CAD build for the part. Positions are in the model's coordinates, mm. A direction names the side the tool comes from. Round coordinates to 2 decimals unless told otherwise and drop trailing zeros. Loops run counter-clockwise (first coordinate to the right, second up) from the corner with the lowest first, then second, coordinate; pieces in that order, holes last.
from build123d import *

# Parameters (mm, degrees)
BASEHEAD_DEPTH  = 7.68
SKETCH3_R       = 6
BASEBODY_DEPTH  = 50
CHAMFER1_SIZE   = 0.947
SLOT_DEPTH      = 60.735123043
SLOT_DEPTH_BACK = 60.735123043
SKETCH5_W       = 3
SKETCH5_H       = 3


with BuildPart() as part:
    # Sketch-BaseHead → BaseHead (new body)
    with BuildSketch(Plane(origin=(0, 0, 0), x_dir=(0, 0, -1), z_dir=(1, 0, 0))):
        Polygon((5.118210136, -8.865), (10.236420273, 0), (5.118210136, 8.865), (-5.118210136, 8.865), (-10.236420273, 0), (-5.118210136, -8.865), align=None)
    extrude(amount=BASEHEAD_DEPTH)

    # Sketch1 → Revolve1 (revolve)
    with BuildSketch(Plane.XY, mode=Mode.PRIVATE) as revolve1_sk:
        Polygon((7.68, 0), (8.18, 0), (8.18, -8.315), (7.68, -8.865), align=None)
    revolve(revolve1_sk.sketch.rotate(Axis((-4.001564945, 0, 0), (1, 0, 0)), 270), axis=Axis((-4.001564945, 0, 0), (1, 0, 0)))

    # Sketch3 → BaseBody (add)
    with BuildSketch(Plane(origin=(8.18, 0, 0), x_dir=(0, 0, -1), z_dir=(1, 0, 0))):
        Circle(SKETCH3_R)
    extrude(amount=BASEBODY_DEPTH)

    # Chamfer1
    chamfer1_edges = [part.edges().sort_by_distance(p)[0] for p in [
        (58.18, 0, 6),
    ]]
    chamfer(chamfer1_edges, length=CHAMFER1_SIZE)

    # Sketch4 → HeadChamfer (revolve, cut)
    with BuildSketch(Plane(origin=(-0.264637255, 0, 5.916896391), x_dir=(0, 0, -1), z_dir=(0, 1, 0))):
        Polygon((16.153316664, -0.264637255), (14.781896391, -0.264637255), (16.153316664, -0.763793413), align=None)
    revolve(axis=Axis((-4.001564945, 0, 0), (1, 0, 0)), mode=Mode.SUBTRACT)

    # Sketch5 → Slot (cut, two sides: drawn at the far end of the back side and taken through both)
    with BuildSketch(Plane(origin=(0, 0, 0), x_dir=(1, 0, 0), z_dir=(0, 1, 0)).offset(-SLOT_DEPTH_BACK)):
        with Locations((1.5, 0)):
            Rectangle(SKETCH5_W, SKETCH5_H)
    extrude(amount=SLOT_DEPTH + SLOT_DEPTH_BACK, mode=Mode.SUBTRACT)


solid = part.part
Item 1: Wall check: L1, parallel to X at y = 3.5, z = -7.25; L2, parallel to X at y = -8, z = 0.25; L3, parallel to Y at x = 26.5, z = 0. Give the ranges that are in metal, low to high.
Verdict:
L1: x = 0 to 8.18
L2: x = 3 to 8.18
L3: y = -6 to 6
Item 2: Mould opens along Z. For faces 1 (the conical face through (0.087, -7.973, -4.392)), 2 (the flat face through (3, 0, 0)), 3 (the flat face through (7.68, 0, 9.2)) say: released by +Z, released by -Z, zero draft, split by the parting line, or undercut.
Verdict:
face 1: released by -Z
face 2: undercut
face 3: zero draft
Item 3: Flat gauge pins, fed straight in: P1, Ø3, axis at x = 6.5, z = 8, coming from the +Y side; P2, Ø0.8, axis at y = 1, z = 9, coming from the +X side; P3, Ø2, axis at y = 6.5, z = 4.5, coming from the +X side; P4, Ø3.5, axis at y = 2.5, z = 0, coming from the -X side. Where does each tip first touch, or does it go through?
Verdict:
P1: stops at y = 6.47
P2: stops at x = 7.87
P3: stops at x = 8.18
P4: stops at x = 0
Item 4: Cut at A-A (x = 10.5). List the corners of the cut face in (y, z).
Verdict:
outline: circle Ø12 at (0, 0)
Item 5: 3-axis set-ups, long thin cutter, end or side, ignore diameter. For faces 4 (the flat face through (1, 0, 1.5)), 5 (the flat face through (7.68, -8, -5)), 6 (the flat face through (7.68, -8, 4.4)): which of +Z, -Z, +X, -X, +Y, -Y reach the whole face in a straight line?
Verdict:
face 4: -X, +Y, -Y
face 5: -Z, +X, -Y
face 6: +Z, +X, -Y
